Geometry check sheet. Reference: the model listing, model coordinates, mm. A direction names the side the tool comes from. Give positions to 0.01 mm unless a question says otherwise; leave off trailing zeros. Write each loop counter-clockwise with the first axis right and the second up, starting at its lowest first coordinate (ties: lowest second). Pieces come first, ordered by that corner, then holes. Notation, with made-up numbers: (-38.75, 52) - (13.25, 52) arc R13 cw to (13.25, 77) - close; hole circle Ø10 at (-2.75, 64). An arc over 180 degrees is marked (long way). Use a Markdown table: item, result.
```python
from build123d import *

# Parameters (mm, degrees)
CUT_EXTRUDE_1_DEPTH = 144.614066163
SKETCH_3_W          = 16
SKETCH_3_H          = 6
CUT_EXTRUDE_2_DEPTH = 147.969384567
CHAMFER_1_SIZE      = 1


with BuildPart() as part:
    # 草图1 → 旋转1 (revolve)
    with BuildSketch(Plane.XY, mode=Mode.PRIVATE) as revolve_1_sk:
        Polygon((35, 0), (100, 0), (100, 15), (60, 15), (60, 40), (35, 40), align=None)
    revolve(revolve_1_sk.sketch.rotate(Axis((0, 0, 0), (0, 1, 0)), 90), axis=Axis((0, 0, 0), (0, 1, 0)))

    # 草图2 → 切除-拉伸1 (cut, through all)
    with BuildSketch(Plane(origin=(0, 15, 0), x_dir=(1, 0, 0), z_dir=(0, 1, 0))):
        with BuildLine():
            ThreePointArc((15.454687812, 87.647890018), (0, 89), (-15.454687812, 87.647890018))
            ThreePointArc((-15.454687812, 87.647890018), (-22.75512399, 77.221786642), (-12.329020614, 69.921350464))
            ThreePointArc((-12.329020614, 69.921350464), (0, 71), (12.329020614, 69.921350464))
            ThreePointArc((12.329020614, 69.921350464), (22.75512399, 77.221786642), (15.454687812, 87.647890018))
        make_face()
        with BuildLine():
            ThreePointArc((69.921350464, -12.329020614), (77.221786642, -22.75512399), (87.647890018, -15.454687812))
            ThreePointArc((87.647890018, -15.454687812), (89, 0), (87.647890018, 15.454687812))
            ThreePointArc((87.647890018, 15.454687812), (77.221786642, 22.75512399), (69.921350464, 12.329020614))
            ThreePointArc((69.921350464, 12.329020614), (71, 0), (69.921350464, -12.329020614))
        make_face()
        with BuildLine():
            ThreePointArc((-12.329020614, -69.921350464), (-22.75512399, -77.221786642), (-15.454687812, -87.647890018))
            ThreePointArc((-15.454687812, -87.647890018), (0, -89), (15.454687812, -87.647890018))
            ThreePointArc((15.454687812, -87.647890018), (22.75512399, -77.221786642), (12.329020614, -69.921350464))
            ThreePointArc((12.329020614, -69.921350464), (0, -71), (-12.329020614, -69.921350464))
        make_face()
        with BuildLine():
            ThreePointArc((-69.921350464, 12.329020614), (-77.221786642, 22.75512399), (-87.647890018, 15.454687812))
            ThreePointArc((-87.647890018, 15.454687812), (-89, 0), (-87.647890018, -15.454687812))
            ThreePointArc((-87.647890018, -15.454687812), (-77.221786642, -22.75512399), (-69.921350464, -12.329020614))
            ThreePointArc((-69.921350464, -12.329020614), (-71, 0), (-69.921350464, 12.329020614))
        make_face()
    extrude(amount=-CUT_EXTRUDE_1_DEPTH, mode=Mode.SUBTRACT)

    # 草图3 → 切除-拉伸2 (cut, through all)
    with BuildSketch(Plane.XZ):
        with Locations((0, 37.073450075)):
            Rectangle(SKETCH_3_W, SKETCH_3_H)
    extrude(amount=-CUT_EXTRUDE_2_DEPTH, mode=Mode.SUBTRACT)

    # 倒角1
    chamfer_1_edges = [part.edges().sort_by_distance(p)[0] for p in [
        (0, 40, 60),
        (0, 15, 100),
        (0, 0, 100),
    ]]
    chamfer(chamfer_1_edges, length=CHAMFER_1_SIZE)


solid = part.part
```
1) Section check A-A on z = 0. Record the boundary of the cut face in (x, y).
Working result:
| item | result |
|---|---|
| outline | (-100, 1) - (-99, 0) - (-89, 0) - (-89, 15) - (-99, 15) - (-100, 14) - close; (-71, 0) - (-35, 0) - (-35, 40) - (-59, 40) - (-60, 39) - (-60, 15) - (-71, 15) - close; (35, 0) - (71, 0) - (71, 15) - (60, 15) - (60, 39) - (59, 40) - (35, 40) - close; (89, 0) - (99, 0) - (100, 1) - (100, 14) - (99, 15) - (89, 15) - close |
2) Material ranges on L1, parallel to X at y = 10.5, z = 0; L2, parallel to X at y = 5.5, z = -19; L3, parallel to X at y = 25, z = 0, recorded low to high. Write a range as from..to.
Working result:
| item | result |
|---|---|
| L1 | x = -100..-89, -71..-35, 35..71, 89..100 |
| L2 | x = -98.18..-86.19, -71.37..-29.39, 29.39..71.37, 86.19..98.18 |
| L3 | x = -60..-35, 35..60 |
3) Set-up check for faces 1 (the flat face through (43, 15, -43)), 2 (the flat face through (-1, 0, 43)), 3 (the cylindrical face through (71, 8, 0)): record each of +Z, -Z, +X, -X, +Y, -Y from which the full face is reachable in a straight line by a thin tool's end or side.
Working result:
| item | result |
|---|---|
| face 1 | +Y |
| face 2 | +Z, -Z, +X, -X, -Y |
| face 3 | +Y, -Y |
4) Depth check by flat-ended pin: P1, Ø3, axis at y = 26, z = 37.5, coming from the -X side; P2, Ø1.5, axis at y = 34, z = -29.5, coming from the +X side; P3, Ø8, axis at y = 13.5, z = 50.5, coming from the -X side; P4, Ø12, axis at x = -7, z = 23, coming from the -Y side. Enter the tip coordinate at first touch or a pass-through.
Working result:
| item | result |
|---|---|
| P1 | stops at x = -48 |
| P2 | stops at x = 52.66 |
| P3 | stops at x = -88.53 |
| P4 | passes through |
5) Section check D-D on y = 7. Record the boundary of the cut face in (x, z), then the cut area to 3 significant figures.
Working result:
| item | result |
|---|---|
| outline | circle Ø200 at (0, 0); hole (-87.65, -15.45) arc R9 ccw to (-69.92, -12.33) arc R71 cw to (-69.92, 12.33) arc R9 ccw to (-87.65, 15.45) arc R89 ccw to start; hole (-15.45, -87.65) arc R89 ccw to (15.45, -87.65) arc R9 ccw to (12.33, -69.92) arc R71 cw to (-12.33, -69.92) arc R9 ccw to start; hole (-15.45, 87.65) arc R9 ccw to (-12.33, 69.92) arc R71 cw to (12.33, 69.92) arc R9 ccw to (15.45, 87.65) arc R89 ccw to start; hole (-8, 34.07) arc R35 ccw (long way) to (8, 34.07) - (8, 40.07) - (-8, 40.07) - close; hole (69.92, -12.33) arc R9 ccw to (87.65, -15.45) arc R89 ccw to (87.65, 15.45) arc R9 ccw to (69.92, 12.33) arc R71 cw to start |
| area | 24,500 mm² |
6) Section check C-C on y = 35.5. Record the boundary of the cut face in (x, z).
Working result:
| item | result |
|---|---|
| outline | circle Ø120 at (0, 0); hole (-8, 34.07) arc R35 ccw (long way) to (8, 34.07) - (8, 40.07) - (-8, 40.07) - close |
7) Section check B-B on x = 0. Record the boundary of the cut face in (y, z).
Working result:
| item | result |
|---|---|
| outline | (0, -99) - (1, -100) - (14, -100) - (15, -99) - (15, -89) - (0, -89) - close; (0, -71) - (15, -71) - (15, -60) - (39, -60) - (40, -59) - (40, -35) - (0, -35) - close; (0, 40.07) - (40, 40.07) - (40, 59) - (39, 60) - (15, 60) - (15, 71) - (0, 71) - close; (0, 89) - (15, 89) - (15, 99) - (14, 100) - (1, 100) - (0, 99) - close |
